Autodesk Inventor part; units mm, degrees
ref_plane "Work Plane1" through (104.775, 0, 0) normal (0, 0, -1) x (1, 0, 0)
ref_plane "YZ Plane" through (0, 0, 0) normal (1, 0, 0) x (0, 1, 0)
ref_plane "XZ Plane" through (0, 0, 0) normal (0, 1, 0) x (-1, 0, 0)
sketch "Skizze1" plane through (0, 0, 0) normal (0, 0, 1) x (1, 0, 0)
  line L0 (16, 0) -> (16, 2)
  line L1 (16, 2) -> (4.58, 2)
  line L2 (4.58, 2) -> (4.1506, 2)
  line L3 (0, 3.765) -> (0, 1.4434)
  line L4 (0, 1.4434) -> (1.5, 1.4434)
  line L5 (1.5, 1.4434) -> (2.3333, 0)
  line L6 (2.3333, 0) -> (16, 0)
  line L7 (0, 3.765) -> (0.715, 3.765)
  line L8 (0.715, 3.765) -> (2.48, 2)
  line L9 (4.1506, 2) -> (2.48, 2)
  line L10 (4.58, 2) -> (2.48, 2) construction
  line L11 (2.48, 2) -> (2.48, 2)
  line L12 (-3.2, 0) -> (19.2, 0)
  line L13 (0, -0.753) -> (0, 4.518)
  dimension "d0" = 16
  dimension "d1" = 11.42
  dimension "d2" = 1.5
  dimension "d3" = 4
  dimension "d6" = 2.48
  dimension "d7" = 45
  dimension "d8" = 2.8868
  dimension "d9" = 60
  dimension "d10" = 7.53
  dimension "d11" = 4
  dimension "d12" = 0.4294
revolve "Körper" add sketch "Skizze1" angle 360 about axis through (2.3333, 0, 0) along (1, 0, 0) contours L6 L5 L4 L3 L7 L8 L9 L2 L1 L0
sketch "Skizze2" plane through (0, 0, 0) normal (-1, 0, 0) x (0, 0, 1)
  circle A0 centre (0, 0) radius 1.4434
  line L0 (0, -5.271) -> (0, 5.271)
  line L1 (-5.271, 0) -> (5.271, 0)
  line L2 (1.4434, 0) -> (0.7217, -1.25)
  line L3 (0.7217, -1.25) -> (-0.7217, -1.25)
  line L4 (-0.7217, -1.25) -> (-1.4434, 0)
  line L5 (-1.4434, 0) -> (-0.7217, 1.25)
  line L6 (-0.7217, 1.25) -> (0.7217, 1.25)
  line L7 (0.7217, 1.25) -> (1.4434, 0)
  point P0 (0, 1.4434)
extrude "Loch" add sketch "Skizze2" against normal up to next contours L7 A0 | A0 L2 | L6 L0 A0 | A0 L0 L3 | L0 L6 A0 | A0 L3 L0 | L4 A0 | A0 L5
thread "Gewinde"
chamfer "Fase1" distance 0.4294 distance2 0.4294 1 edges at (16, -2, 0) measured on face at (16, 0.2227, -0.5871)
ref_plane "Work Plane1" through (104.775, 0, 0) normal (0, 0, -1) x (1, 0, 0)
equation "\"d15\" = GEL"
equation "\"d17\" = -0.5 * SPD + 0.5 * GD"
equation "\"d18\" = GUL"
equation "\"d0\" = NLG"
equation "\"d1\" = GEL"
equation "\"d2\" = INTI"
equation "\"d3\" = GD"
equation "\"d6\" = KOH"
equation "\"d7\" = 0.5 * SEWI"
equation "\"d8\" = 1.1547 * SW"
equation "\"d10\" = KOD"
equation "\"d11\" = BDM"
equation "\"d12\" = GAL"
equation "\"NLG\" = 16"
equation "\"INTI\" = 1.5"
equation "\"GEL\" = 11.42"
equation "\"GAL\" = 0.61345 * PTC"
equation "\"KOH\" = 2.48"
equation "\"KOD\" = 7.53"
equation "\"GUL\" = 0.61345 * PTC"
equation "\"SPD\" = NND - 1.2269 * PTC"
equation "\"BDM\" = NND"
equation "\"GD\" = NND"
equation "\"SEWI\" = 90deg"
equation "\"SW\" = 2.5"
equation "\"TOA\" = 30deg"
equation "\"GD1\" = THREADDIA - 1.2269 * PTC"
equation "\"EPV\" = 4.58"
equation "\"THREADDIA\" = 4"
equation "\"PTC\" = 0.7"
equation "\"NND\" = 4"
equation "\"E0\" = 2.89"
properties part number "ISO 10642  - M4  x  16" material "Stahl"
Work out the finished part from the listing and answer in its coordinate system (mm). A direction names the side the tool comes from. Give positions to 0.01 mm unless a question says otherwise; leave off trailing zeros. Loops run counter-clockwise (first coordinate to the right, second up) from the corner with the lowest first, then second, coordinate; pieces in that order, holes last. Notation, with made-up numbers: (55, 67) - (60, 67) arc R7 cw to (60, 71) - close; hole circle Ø8 at (79.25, 29). An arc over 180 degrees is marked (long way). One line per question, with ' | ' between items.
(1) A tool of negligible diameter and unlimited length cuts with its end or side. For faces 4 (the face through (0.363, -0.49, 3.733)), 5 (the face through (1, -1.25, 0)), from which of +Z, -Z, +X, -X, +Y, -Y can it reach the whole face along a straight path? Write none if from no direction.
Recorded:
face 4: +X, -X | face 5: -X
(2) Each of these flat-tipped pins is pushed along its axis until it touches: pin 1 Ø1.5 at (x, z) = (8.5, 2.5) entering from +Y; pin 2 Ø4 at (x, z) = (7.5, 1) entering from -Y; pin 3 Ø4 at (x, z) = (5, 3) entering from -Y. Where does it stop, or does it pass through?
Recorded:
pin 1: stops at y = 0.97 | pin 2: stops at y = -2 | pin 3: stops at y = -1.73
(3) Straight lines are drawn through the part: probe 1 along Z at (x, y) = (13.25, 0); probe 2 along Y at (x, z) = (13, 0.75); probe 3 along Y at (x, z) = (10, 1). For each, find the intervals that lie inside material, in ascending order.
Recorded:
probe 1: z = -2 to 2 | probe 2: y = -1.85 to 1.85 | probe 3: y = -1.73 to 1.73
(4) The mould has two halves that part along Z. Classify faces 1 (the face through (9, 0, 2)), 2 (the face through (0, 0, 2)), 3 (the face through (2.28, 0.09, -0.03)): +Z half, -Z half, draft (parallel to the pull), parting line (faces both ways), or undercut.
Recorded:
face 1: parting line | face 2: draft | face 3: undercut
(5) The part is cut by section A-A (x = 6.5). Write down the section's boundary in (y, z).
Recorded:
outline: circle Ø4 at (0, 0)
